For this review, take the finished solid that the model builds, in its own axes (mm). A direction names the side the tool comes from. Give positions to 0.01 mm unless a question says otherwise; leave off trailing zeros. Write each loop counter-clockwise with the first axis right and the second up, starting at its lowest first coordinate (ties: lowest second). Pieces come first, ordered by that corner, then holes. Notation, with made-up numbers: (42, 82.25) -> (54, 82.25) arc R26 cw to (54, 118.25) -> close; hole circle Ø4 at (9.5, -11). An arc over 180 degrees is marked (long way). Return JSON: item names as keys, results as strings.
Autodesk Inventor part; units mm, degrees
ref_plane "YZ Plane" through (0, 0, 0) normal (1, 0, 0) x (0, 1, 0)
ref_plane "XZ Plane" through (0, 0, 0) normal (0, 1, 0) x (-1, 0, 0)
ref_plane "XY Plane" through (0, 0, 0) normal (0, 0, 1) x (1, 0, 0)
sketch "Sketch1" plane through (0, 0, 0) normal (0, 1, 0) x (-1, 0, 0)
  circle A0 centre (0, 0) radius 127
  dimension "d0" = 254
extrude "Extrusion1" add sketch "Sketch1" along normal mid plane 12.7
sketch "Sketch2" plane through (0, 6.35, 0) normal (0, 1, 0) x (1, 0, 0)
  circle A0 centre (0, 0) radius 101.6
  dimension "d3" = 203.2
extrude "Extrusion2" cut sketch "Sketch2" against normal blind 1.5875
mirror "Mirror1" about plane through (0, 0, 0) normal (0, 1, 0) of "Extrusion2"
properties part number "Chip, Simplified" material "Polycarbonate, Clear"
1. For faces 1 (the flat face through (1, -4.762, -1)), 2 (the flat face through (-1, 4.762, -1)), 3 (the flat face through (57, 6.35, 85)), list the 3-axis set-ups (+Z, -Z, +X, -X, +Y, -Y) from which the entire face can be reached by the end or side of a thin tool; tool diameter is ignored.
Results found:
{"face 1": "-Y", "face 2": "+Y", "face 3": "+Z, -Z, +X, -X, +Y"}
2. Add section B-B, the plane z = 0. State the section outline as (x, y) points.
Results found:
{"outline": "(-127, -6.35) -> (-101.6, -6.35) -> (-101.6, -4.76) -> (101.6, -4.76) -> (101.6, -6.35) -> (127, -6.35) -> (127, 6.35) -> (101.6, 6.35) -> (101.6, 4.76) -> (-101.6, 4.76) -> (-101.6, 6.35) -> (-127, 6.35) -> close"}
3. Add section C-C, the plane y = 1. State the section outline as (x, z) points, plus the area to 3 significant figures.
Results found:
{"outline": "circle Ø254 at (0, 0)", "area": "50,700 mm²"}
4. The part is to be moulded in two halves that separate along X. For faces 4 (the cylindrical face through (27.53, -0.09, 123.98)), 5 (the cylindrical face through (-22.025, -5.567, -99.184)), 6 (the flat face through (57, -6.35, 85)), say which applies: +X half, -X half, draft (parallel to the pull), parting line (faces both ways), or undercut.
Results found:
{"face 4": "parting line", "face 5": "undercut", "face 6": "draft"}
5. Add section D-D, the plane x = 105. State the section outline as (y, z) points.
Results found:
{"outline": "(-6.35, -71.44) -> (6.35, -71.44) -> (6.35, 71.44) -> (-6.35, 71.44) -> close"}
6. Add section A-A, the plane x = 0. State the section outline as (y, z) points, plus the area to 3 significant figures.
Results found:
{"outline": "(-6.35, -127) -> (6.35, -127) -> (6.35, -101.6) -> (4.76, -101.6) -> (4.76, 101.6) -> (6.35, 101.6) -> (6.35, 127) -> (-6.35, 127) -> (-6.35, 101.6) -> (-4.76, 101.6) -> (-4.76, -101.6) -> (-6.35, -101.6) -> close", "area": "2,580 mm²"}
7. For pin 1 (6 mm diameter, centred on x = -65, z = 38.5, fed in from -Y); pin 2 (2 mm diameter, centred on y = 1, z = -70, fed in from -X); pin 3 (12 mm diameter, centred on x = 46.5, z = -66.5, fed in from +Y), all flat-tipped, find the tip position at first contact; note any pin that passes through.
Results found:
{"pin 1": "stops at y = -4.76", "pin 2": "stops at x = -106.62", "pin 3": "stops at y = 4.76"}
8. To check wall thickness, follow probe 1 along Z at (x, y) = (0, 5.55); probe 2 along Y at (x, z) = (49, 46); probe 3 along Z at (x, y) = (1, 1). State the ranges of each line that lie inside material, in increasing order.
Results found:
{"probe 1": "z = -127 to -101.6, 101.6 to 127", "probe 2": "y = -4.76 to 4.76", "probe 3": "z = -127 to 127"}
